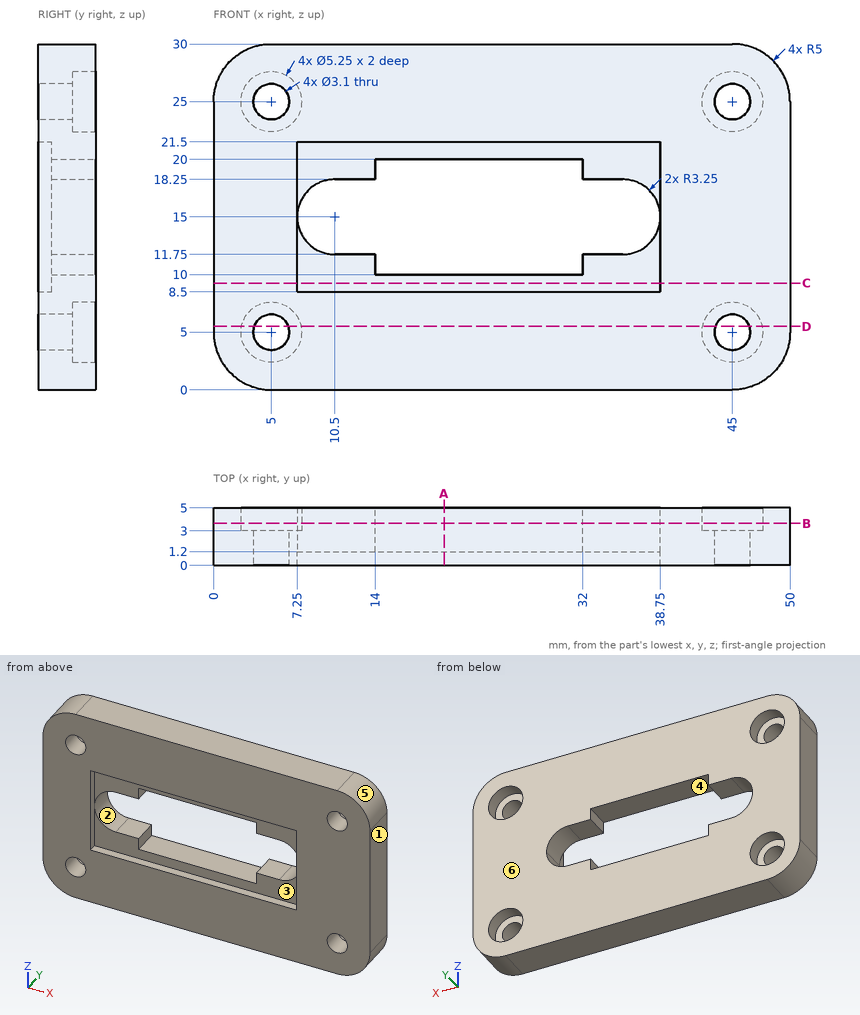
Part print with two shaded views. Sizes in mm from the minimum x, y, z corner. A direction names the side the tool comes from. Coordinates: 2 decimals unless noted, no trailing zeros. Write each loop counter-clockwise with the first axis right and the second up, starting at its lowest first coordinate (ties: lowest second). Pieces come first, ordered by that corner, then holes.
1. Drill centre lines: probe 1 along X at (y, z) = (4.5, 5) (3 decimals); probe 2 along X at (y, z) = (1.8, 5); probe 3 along Z at (x, y) = (45, 3.95) (3 decimals). Where is each one in solid material? Low to high.
Answer block:
probe 1: x = 0 to 2.375, 7.625 to 42.375, 47.625 to 50
probe 2: x = 0 to 3.45, 6.55 to 43.45, 46.55 to 50
probe 3: z = 0 to 2.375, 7.625 to 22.375, 27.625 to 30
2. Drop flat-ended pins along their axis: pin 1 (3 mm diameter, centred on x = 32, y = 2, fed in from -Z); pin 2 (6 mm diameter, centred on x = 29.5, z = 13.5, fed in from +Y); pin 3 (4 mm diameter, centred on x = 5, z = 5.5, fed in from +Y). Give the stop position or say it passes through.
Answer block:
pin 1: stops at z = 0
pin 2: passes through
pin 3: stops at y = 3
3. Band-saw the part on B-B, the plane y = 3.65. Give the cut face in (x, z) (3 decimals), and give its area (3 significant figures).
Answer block:
outline: (0, 5) arc R5 ccw to (5, 0) - (45, 0) arc R5 ccw to (50, 5) - (50, 25) arc R5 ccw to (45, 30) - (5, 30) arc R5 ccw to (0, 25) - close; hole circle Ø5.25 at (5, 5); hole circle Ø5.25 at (5, 25); hole (10.5, 11.75) - (14, 11.75) - (14, 10) - (32, 10) - (32, 11.75) - (35.5, 11.75) arc R3.25 ccw to (35.5, 18.25) - (32, 18.25) - (32, 20) - (14, 20) - (14, 18.25) - (10.5, 18.25) arc R3.25 ccw to start; hole circle Ø5.25 at (45, 5); hole circle Ø5.25 at (45, 25)
area: 1,130 mm2
4. Band-saw the part on A-A, the plane x = 20. Give the cut face in (y, z).
Answer block:
outline: (0, 0) - (5, 0) - (5, 10) - (1.2, 10) - (1.2, 8.5) - (0, 8.5) - close; (0, 21.5) - (1.2, 21.5) - (1.2, 20) - (5, 20) - (5, 30) - (0, 30) - close
5. Band-saw the part on C-C, the plane z = 9.25. Give the cut face in (x, y), and give its area (3 significant figures).
Answer block:
outline: (0, 0) - (7.25, 0) - (7.25, 1.2) - (38.75, 1.2) - (38.75, 0) - (50, 0) - (50, 5) - (0, 5) - close
area: 212 mm2
6. 3-axis set-ups, long thin cutter, end or side, ignore diameter. For the marked faces 1, 2 and 3: which of +Z, -Z, +X, -X, +Y, -Y reach the whole face in a straight line?
Answer block:
face 1: +Z, -Z, +X, +Y, -Y
face 2: +Y, -Y
face 3: -Y
7. Band-saw the part on D-D, the plane z = 5.5. Give the cut face in (x, y), and give its area (3 significant figures).
Answer block:
outline: (0, 0) - (3.53, 0) - (3.53, 3) - (2.42, 3) - (2.42, 5) - (0, 5) - close; (6.47, 0) - (43.53, 0) - (43.53, 3) - (42.42, 3) - (42.42, 5) - (7.58, 5) - (7.58, 3) - (6.47, 3) - close; (46.47, 0) - (50, 0) - (50, 5) - (47.58, 5) - (47.58, 3) - (46.47, 3) - close
area: 212 mm2
8. Pull direction Z, two halves, no side cores. Call the marked faces 4, 5 and 6: released by +Z, released by -Z, zero draft, split by the parting line, or undercut.
Answer block:
face 4: undercut
face 5: released by +Z
face 6: zero draft
